Part model, mm, in its own coordinate system. A direction names the side the tool comes from. Coordinates: 2 decimals unless noted, no trailing zeros. Write each loop counter-clockwise with the first axis right and the second up, starting at its lowest first coordinate (ties: lowest second). Pieces come first, ordered by that corner, then holes. Notation, with made-up numbers: M -34.5,2.25 L -16.5,2.25 A17 ccw -16.5,24.25 Z; hole C 13.5,40.25 d4. An arc over 180 degrees is marked long. Use a Markdown table: item, result. Add a question column.
Q1. Slice it at D-D on x = 8. Write the cut outline in (y, z).
Q2. Tool access for faces 1 (the flat face through (-19.001, 1, 0)), 2 (the flat face through (0, 1, -2.5)), 3 (the flat face through (2.5, 1, 0)), 4 (the flat face through (0, 2.5, 0)), 5 (the flat face through (16, 1, 2.5)): list every direction of +Z, -Z, +X, -X, +Y, -Y with a clear straight run to the whole face (end or side of a thin tool).
Q3. Pin check, flat tips, straight feed: pin 1 Ø0.6 at (x, y) = (-1, 1.5) entering from -Z; pin 2 Ø0.6 at (y, z) = (1.5, 0) entering from -X. Stop position of each tip, or through.
Q4. Mould opens along X. For faces 6 (the flat face through (-17, 1, 2.5)), 7 (the flat face through (19.001, 1, 0)), 8 (the flat face through (-14.001, 1, 0)), 9 (the flat face through (14.001, 1, 0)) say: released by +X, released by -X, zero draft, split by the parting line, or undercut.
Q5. Slice it at A-A on z = -0.5. Write the cut outline in (x, y), then the cut area to 3 significant figures.
Q6. Slice it at B-B on y = 1.1. Write the cut outline in (x, z), then the cut area to 3 significant figures.
Q7. Wall check: L1, parallel to X at y = 2.2, z = -2; L2, parallel to Z at x = 1.5, y = 2.4; L3, parallel to Y at x = 13, z = 3. Give the ranges that are in metal, low to high. Write a range as from..to.
Q8. Slice it at C-C on x = 15. Write the cut outline in (y, z).
from build123d import *

# Parameters (mm, degrees)
SKETCH1_W            = 50
SKETCH1_H            = 10
BOSS_EXTRUDE1_DEPTH  = 0.5
SKETCH12_W           = 5
SKETCH12_H           = 5
BOSS_EXTRUDE8_DEPTH  = 2
SKETCH13_W           = 5
SKETCH13_H           = 5
BOSS_EXTRUDE9_DEPTH  = 2
SKETCH14_W           = 5
SKETCH14_H           = 5
BOSS_EXTRUDE10_DEPTH = 2


with BuildPart() as part:
    # Sketch1 → Boss-Extrude1 (new body)
    with BuildSketch(Plane(origin=(0, 0, 0), x_dir=(1, 0, 0), z_dir=(0, 1, 0))):
        Rectangle(SKETCH1_W, SKETCH1_H)
    extrude(amount=BOSS_EXTRUDE1_DEPTH)

    # Sketch12 → Boss-Extrude8 (add)
    with BuildSketch(Plane(origin=(0, 0.5, 0), x_dir=(1, 0, 0), z_dir=(0, 1, 0))):
        with Locations((-16.500638267, 0)):
            Rectangle(SKETCH12_W, SKETCH12_H)
    extrude(amount=BOSS_EXTRUDE8_DEPTH)

    # Sketch13 → Boss-Extrude9 (add)
    with BuildSketch(Plane(origin=(0, 0.5, 0), x_dir=(1, 0, 0), z_dir=(0, 1, 0))):
        Rectangle(SKETCH13_W, SKETCH13_H)
    extrude(amount=BOSS_EXTRUDE9_DEPTH)

    # Sketch14 → Boss-Extrude10 (add)
    with BuildSketch(Plane(origin=(0, 0.5, 0), x_dir=(1, 0, 0), z_dir=(0, 1, 0))):
        with Locations((16.500638267, 0)):
            Rectangle(SKETCH14_W, SKETCH14_H)
    extrude(amount=BOSS_EXTRUDE10_DEPTH)


solid = part.part
Recorded:
| question | item | result |
|---|---|---|
| 1 | outline | M 0,-5 L 0.5,-5 L 0.5,5 L 0,5 Z |
| 2 | face 1 | +Z, -Z, -X, +Y |
| 2 | face 2 | -Z, +X, -X, +Y |
| 2 | face 3 | +Z, -Z, +Y |
| 2 | face 4 | +Z, -Z, +X, -X, +Y |
| 2 | face 5 | +Z, +X, -X, +Y |
| 3 | pin 1 | z = -2.5 |
| 3 | pin 2 | x = -19 |
| 4 | face 6 | zero draft |
| 4 | face 7 | released by +X |
| 4 | face 8 | undercut |
| 4 | face 9 | undercut |
| 5 | outline | M -25,0 L 25,0 L 25,0.5 L 19,0.5 L 19,2.5 L 14,2.5 L 14,0.5 L 2.5,0.5 L 2.5,2.5 L -2.5,2.5 L -2.5,0.5 L -14,0.5 L -14,2.5 L -19,2.5 L -19,0.5 L -25,0.5 Z |
| 5 | area | 55.0 mm² |
| 6 | outline | M -19,-2.5 L -14,-2.5 L -14,2.5 L -19,2.5 Z; M -2.5,-2.5 L 2.5,-2.5 L 2.5,2.5 L -2.5,2.5 Z; M 14,-2.5 L 19,-2.5 L 19,2.5 L 14,2.5 Z |
| 6 | area | 75.0 mm² |
| 7 | L1 | -19..-14, -2.5..2.5, 14..19 |
| 7 | L2 | -2.5..2.5 |
| 7 | L3 | 0..0.5 |
| 8 | outline | M 0,-5 L 0.5,-5 L 0.5,-2.5 L 2.5,-2.5 L 2.5,2.5 L 0.5,2.5 L 0.5,5 L 0,5 Z |
